Geometry: final body of the model. Coordinates: model frame, mm. Give positions to 0.01 mm unless a question says otherwise; leave off trailing zeros. Order: outer loops, then holes, each group sorted by start corner. A loop starts at its lowest first (then second) coordinate and runs counter-clockwise, first axis right, second up. Notation, with made-up numbers: M 85.5,18.5 L 115.5,18.5 A8 ccw 115.5,32.5 Z; hole C 77,60.25 d7. An arc over 180 degrees is marked long. Use CSV: the item, a comma, the result in double quotes.
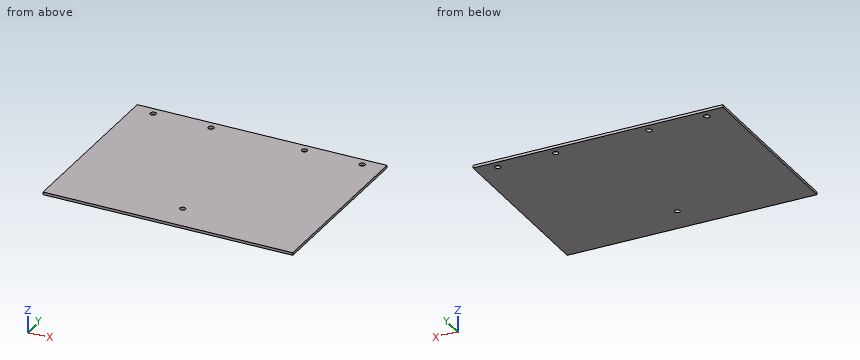
```python
from build123d import *

# Parameters (mm, degrees)
SKETCH_1_W          = 190
SKETCH_1_H          = 140
EXTRUDE_1_DEPTH     = 2
SKETCH_2_R          = 2.15
SKETCH_2_R_2        = 2.2
CUT_EXTRUDE_1_DEPTH = 10
SKETCH_3_R          = 2.1
CUT_EXTRUDE_2_DEPTH = 10


with BuildPart() as part:
    # ｽｹｯﾁ1 → ﾎﾞｽ - 押し出し1 (new body)
    with BuildSketch(Plane.XY):
        Rectangle(SKETCH_1_W, SKETCH_1_H)
    extrude(amount=EXTRUDE_1_DEPTH)

    # ｽｹｯﾁ2 → ｶｯﾄ - 押し出し1 (cut)
    with BuildSketch(Plane.XY.offset(2)):
        with Locations((35.5, 63.5)):
            Circle(SKETCH_2_R)
        with Locations((79.5, 63.5)):
            Circle(SKETCH_2_R)
        with Locations((-35.5, 63.5)):
            Circle(SKETCH_2_R_2)
        with Locations((-79.5, 63.5)):
            Circle(SKETCH_2_R_2)
    extrude(amount=-CUT_EXTRUDE_1_DEPTH, mode=Mode.SUBTRACT)

    # ｽｹｯﾁ3 → ｶｯﾄ - 押し出し2 (cut)
    with BuildSketch(Plane.XY.offset(2)):
        with Locations((0, -48)):
            Circle(SKETCH_3_R)
    extrude(amount=-CUT_EXTRUDE_2_DEPTH, mode=Mode.SUBTRACT)


solid = part.part
```
1. Pin query (flat end, axial travel): pin 1 Ø4 at (x, y) = (79.5, 63.5) entering from +Z. Return the tip coordinate at first contact, or that it passes through.
Answer:
pin 1,"through"
2. Line query: line 1 (Y direction, x = 35.5, z = 1.55); line 2 (Y direction, x = -79.5, z = 1.1). Output: solid intervals per line, ascending.
Answer:
line 1,"-70 to 61.35, 65.65 to 70"
line 2,"-70 to 61.3, 65.7 to 70"
3. Section A-A, the plane x = -35.5. Return the cut outline in (y, z).
Answer:
outline,"M -70,0 L 61.3,0 L 61.3,2 L -70,2 Z; M 65.7,0 L 70,0 L 70,2 L 65.7,2 Z"
4. Section B-B, the plane y = -48. Return the cut outline in (x, z), plus the area to 3 significant figures.
Answer:
outline,"M -95,0 L -2.1,0 L -2.1,2 L -95,2 Z; M 2.1,0 L 95,0 L 95,2 L 2.1,2 Z"
area,"372 mm2"
5. Section C-C, the plane y = 63.5. Return the cut outline in (x, z), plus the area to 3 significant figures.
Answer:
outline,"M -95,0 L -81.7,0 L -81.7,2 L -95,2 Z; M -77.3,0 L -37.7,0 L -37.7,2 L -77.3,2 Z; M -33.3,0 L 33.35,0 L 33.35,2 L -33.3,2 Z; M 37.65,0 L 77.35,0 L 77.35,2 L 37.65,2 Z; M 81.65,0 L 95,0 L 95,2 L 81.65,2 Z"
area,"345 mm2"
